For this review, use the dimensioned drawing (mm, ordinates from the lowest corner) and the shaded views. A direction names the side the tool comes from. Give positions to 0.01 mm unless a question says otherwise; leave off trailing zeros. Loops run counter-clockwise (first coordinate to the right, second up) from the corner with the lowest first, then second, coordinate; pieces in that order, holes last. Notation, with made-up numbers: M 30.5,-23 L 39.5,-23 A14 ccw 39.5,-11 Z; hole C 7.25,-21 d11. An arc over 180 degrees is marked long. Use CSV: the item, a comma, the result in double quotes.
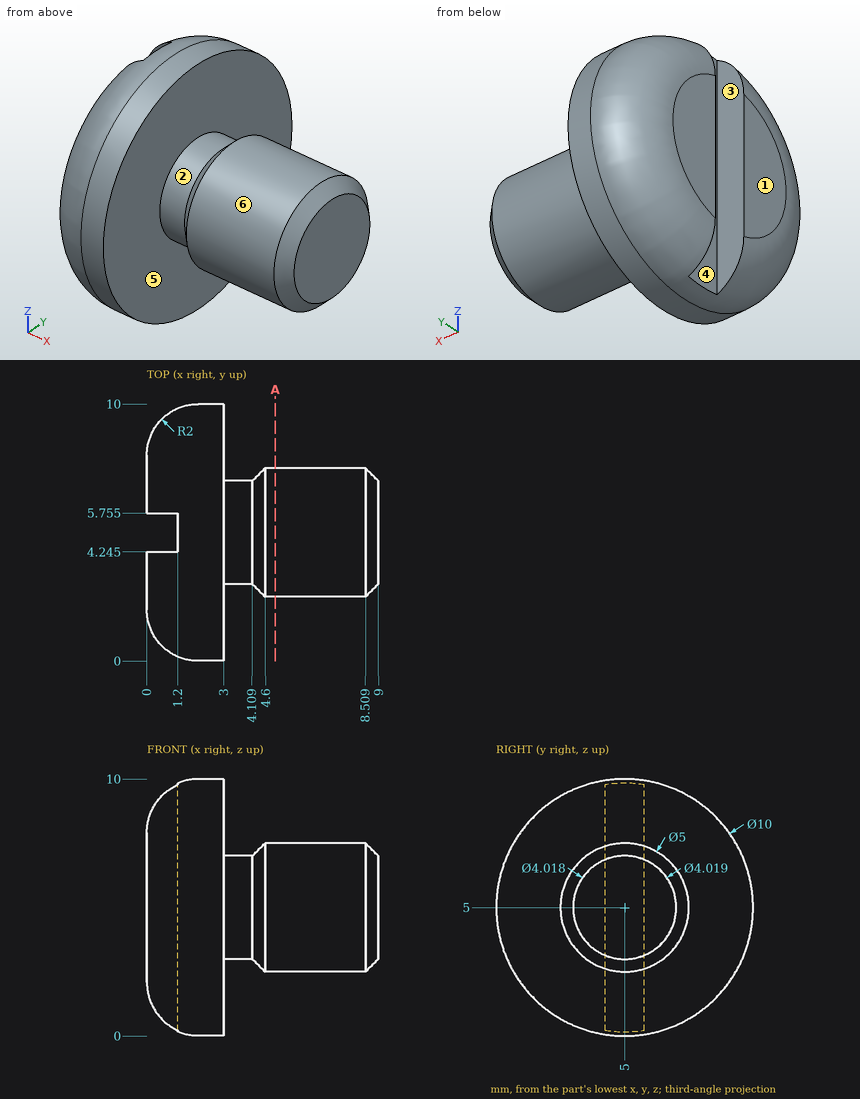
(1) Wall thickness on line 1 along X through (y, z) = (5, 4.75); line 2 along Y through (x, z) = (1, 5.5) (1 decimal); line 3 along Z through (x, y) = (6.75, 4.5): over which ranges is each line inside the solid? List them lowest first. Write a range as [from, to].
A:
line 1,"[1.2, 9]"
line 2,"[0.3, 4.2], [5.8, 9.7]"
line 3,"[2.55, 7.45]"
(2) We need section A-A on x = 5. State the section outline as (y, z) points.
A:
outline,"C 5,5 d5"
(3) Machinability: for the marked faces 1, 2 and 3, which of the approach directions +Z, -Z, +X, -X, +Y, -Y give a long, thin tool a straight path to every point of the face, cutting with its end or side? Answer none if there is none.
A:
face 1,"+Z, -Z, -X, +Y, -Y"
face 2,"none"
face 3,"+Z, -Z, -X"
(4) Clearance check with flat-ended pins moving along their axes: P1, Ø2, axis at x = 5, z = 6.5, coming from the +Y side; P2, Ø3, axis at x = 5.5, y = 2, coming from the -Z side; P3, Ø4, axis at x = 7.5, z = 4, coming from the -Y side; P4, Ø3, axis at y = 7, z = 6, coming from the +X side. State where each tip first meets the part, or that it passes through.
A:
P1,"y = 7.45"
P2,"z = 3"
P3,"y = 2.5"
P4,"x = 9"
(5) The part is to be moulded in two halves that separate along Y. For the marked faces 4, 5 and 6, say which applies: released by +Y, released by -Y, zero draft, split by the parting line, or undercut.
A:
face 4,"undercut"
face 5,"zero draft"
face 6,"split by the parting line"
